Here's how the part is built. I have some questions about the finished solid (model axes, mm). Round coordinates to 2 decimals unless told otherwise and drop trailing zeros. Loops run counter-clockwise (first coordinate to the right, second up) from the corner with the lowest first, then second, coordinate; pieces in that order, holes last. Notation, with made-up numbers: (-25.5, 64.25) - (13.5, 64.25) arc R25 cw to (13.5, 100.25) - close; hole circle Ø6 at (-40, -15.75). An arc over 180 degrees is marked (long way). Answer as a JSON object with one key per item and string values. Group by question number.
1) I want a section at D-D, the plane y = 9. Please give me the cut outline in (x, z) (3 decimals), then the cut area to 3 significant figures.
2) I want a section at A-A, the plane y = 3. Please give me the cut outline in (x, z) (3 decimals).
3) If we mould it in two halves opening along Z, with no side actions, what happens to faces 1 (the face through (15, 5, 0)), 2 (the face through (0, 5, 24)), 3 (the face through (14.79, 6.996, 40.934))? For each: pulls with the +Z half, pulls with the -Z half, needs draft (parallel to the pull), parting line crosses it, or undercut.
4) If I drill on line 1 along Z through (x, y) = (10.25, 8.5); line 2 along Y through (x, z) = (9.25, 40.5); line 3 along Y through (x, z) = (13.75, 39), over which ranges is the centre line in solid material (lowest first)? Write a range as [from, to].
5) I want a section at C-C, the plane z = 14.5. Please give me the cut outline in (x, y), then the cut area to 3 significant figures.
6) I want a section at B-B, the plane x = 24. Please give me the cut outline in (y, z) (3 decimals), then the cut area to 3 significant figures.
7) Will these pins go through, and if not, where does the flat tip stop? P1, Ø6.5, axis at x = 24, z = 31.995, coming from the -Y side; P2, Ø3.5, axis at x = 24, z = 16.005, coming from the -Y side.
from build123d import *

# Parameters (mm, degrees)
SKETCH_1_W          = 30
SKETCH_1_H          = 10
EXTRUDE_1_DEPTH     = 48
SKETCH_3_R          = 3.005
CUT_EXTRUDE_1_DEPTH = 48
SKETCH_4_R          = 2
CUT_EXTRUDE_2_DEPTH = 58.480431453


with BuildPart() as part:
    # 草图1 → 凸台-拉伸1 (new body)
    with BuildSketch(Plane.XY):
        with Locations((15, 5)):
            Rectangle(SKETCH_1_W, SKETCH_1_H)
    extrude(amount=EXTRUDE_1_DEPTH)

    # 草图3 → 切除-拉伸1 (cut)
    with BuildSketch(Plane.ZY):
        with Locations((7, 10)):
            Circle(SKETCH_3_R)
        with Locations((41, 10)):
            Circle(SKETCH_3_R)
    extrude(amount=-CUT_EXTRUDE_1_DEPTH, mode=Mode.SUBTRACT)

    # 草图4 → 切除-拉伸2 (cut, through all)
    with BuildSketch(Plane(origin=(0, 10, 0), x_dir=(1, 0, 0), z_dir=(0, 1, 0))):
        with Locations(Location((24, -31.995, 0), (0, 0, 270))):
            Circle(SKETCH_4_R)
        with Locations(Location((6, -31.995, 0), (0, 0, 270))):
            Circle(SKETCH_4_R)
        with Locations(Location((24, -16.005, 0), (0, 0, 270))):
            Circle(SKETCH_4_R)
        with Locations(Location((6, -16.005, 0), (0, 0, 270))):
            Circle(SKETCH_4_R)
    extrude(amount=-CUT_EXTRUDE_2_DEPTH, mode=Mode.SUBTRACT)


solid = part.part
Outcome:
{
 "1": {"outline": "(0, 0) - (30, 0) - (30, 4.166) - (0, 4.166) - close; (0, 9.834) - (30, 9.834) - (30, 38.166) - (0, 38.166) - close; (0, 43.834) - (30, 43.834) - (30, 48) - (0, 48) - close; hole circle Ø4 at (6, 16.005); hole circle Ø4 at (6, 31.995); hole circle Ø4 at (24, 16.005); hole circle Ø4 at (24, 31.995)", "area": "1,050 mm^2"},
 "2": {"outline": "(0, 0) - (30, 0) - (30, 48) - (0, 48) - close; hole circle Ø4 at (6, 16.005); hole circle Ø4 at (6, 31.995); hole circle Ø4 at (24, 16.005); hole circle Ø4 at (24, 31.995)"},
 "3": {"face 1": "pulls with the -Z half", "face 2": "needs draft", "face 3": "undercut"},
 "4": {"line 1": "[0, 4.4], [9.6, 38.4], [43.6, 48]", "line 2": "[0, 7.04]", "line 3": "[0, 7.76]"},
 "5": {"outline": "(0, 0) - (4.68, 0) - (4.68, 10) - (0, 10) - close; (7.32, 0) - (22.68, 0) - (22.68, 10) - (7.32, 10) - close; (25.32, 0) - (30, 0) - (30, 10) - (25.32, 10) - close", "area": "247 mm^2"},
 "6": {"outline": "(0, 0) - (10, 0) - (10, 3.995) arc R3.005 cw to (10, 10.005) - (10, 14.005) - (0, 14.005) - close; (0, 18.005) - (10, 18.005) - (10, 29.995) - (0, 29.995) - close; (0, 33.995) - (10, 33.995) - (10, 37.995) arc R3.005 cw to (10, 44.005) - (10, 48) - (0, 48) - close", "area": "372 mm^2"},
 "7": {"P1": "y = 0", "P2": "through"}
}
